from build123d import *

# Parameters (mm, degrees)
SKETCH1_R                = 5
BOSS_EXTRUDE1_DEPTH      = 10
BOSS_EXTRUDE2_DEPTH      = 30
BOSS_EXTRUDE2_DEPTH_BACK = 10
SKETCH2_W                = 140
SKETCH2_H                = 10
CUT_EXTRUDE1_DEPTH       = 30
FILLET1_R                = 10


with BuildPart() as part:
    # Sketch1 → Boss-Extrude1 (new body)
    with BuildSketch(Plane(origin=(0, 0, 0), x_dir=(1, 0, 0), z_dir=(0, 1, 0))):
        with BuildLine():
            Line((0, 0), (0, 35))
            ThreePointArc((0, 35), (4.679111138, 47.855752194), (16.527036447, 54.69615506))
            Line((16.527036447, 54.69615506), (86.139090058, 66.970638294))
            ThreePointArc((86.139090058, 66.970638294), (98.064418846, 65.400638975), (106.932561687, 57.274483234))
            Line((106.932561687, 57.274483234), (140, 0))
            Line((140, 0), (0, 0))
        make_face()
        with Locations(Location((20, 35, 0), (0, 0, 270))):
            Circle(SKETCH1_R, mode=Mode.SUBTRACT)
        with Locations(Location((89.612053611, 47.274483234, 0), (0, 0, 270))):
            Circle(SKETCH1_R, mode=Mode.SUBTRACT)
        with BuildLine():
            Line((122.679491924, 10), (10, 10))
            Line((10, 10), (10, 17.962162855))
            ThreePointArc((10, 17.962162855), (12.003313152, 21.964645576), (16.407947174, 22.759837787))
            ThreePointArc((16.407947174, 22.759837787), (29.771929506, 26.800377555), (31.430453218, 40.662963335))
            ThreePointArc((31.430453218, 40.662963335), (31.448708001, 45.138764747), (35.042512339, 47.806666902))
            Line((35.042512339, 47.806666902), (69.815261378, 53.938040751))
            ThreePointArc((69.815261378, 53.938040751), (74.069509797, 52.692990027), (75.66252141, 48.556434103))
            ThreePointArc((75.66252141, 48.556434103), (83.691884517, 34.57863964), (99.560671411, 37.412543742))
            ThreePointArc((99.560671411, 37.412543742), (103.753425217, 38.851152942), (107.441767577, 36.39251276))
            Line((107.441767577, 36.39251276), (122.679491924, 10))
        make_face(mode=Mode.SUBTRACT)
    extrude(amount=BOSS_EXTRUDE1_DEPTH)

    # Sketch2 → Boss-Extrude2 (add, two sides: drawn at the far end of the back side and taken through both)
    with BuildSketch(Plane(origin=(0, 10, 0), x_dir=(1, 0, 0), z_dir=(0, 1, 0)).offset(-BOSS_EXTRUDE2_DEPTH_BACK)):
        with Locations((70, -5)):
            Rectangle(SKETCH2_W, SKETCH2_H)
    extrude(amount=BOSS_EXTRUDE2_DEPTH + BOSS_EXTRUDE2_DEPTH_BACK)

    # Sketch3 → Cut-Extrude1 (cut)
    with BuildSketch(Plane(origin=(0, 0, 0), x_dir=(-1, 0, 0), z_dir=(0, 0, -1))):
        with BuildLine():
            Line((-125, 31), (-75, 31))
            ThreePointArc((-75, 31), (-69, 25), (-75, 19))
            Line((-75, 19), (-125, 19))
            ThreePointArc((-125, 19), (-131, 25), (-125, 31))
        make_face()
        with BuildLine():
            Line((-55, 31), (-20, 31))
            ThreePointArc((-20, 31), (-14, 25), (-20, 19))
            Line((-20, 19), (-55, 19))
            ThreePointArc((-55, 19), (-61, 25), (-55, 31))
        make_face()
    extrude(amount=-CUT_EXTRUDE1_DEPTH, mode=Mode.SUBTRACT)

    # Fillet1
    fillet1_edges = [part.edges().sort_by_distance(p)[0] for p in [
        (0, 40, 5),
        (140, 40, 5),
    ]]
    fillet(fillet1_edges, radius=FILLET1_R)


solid = part.part
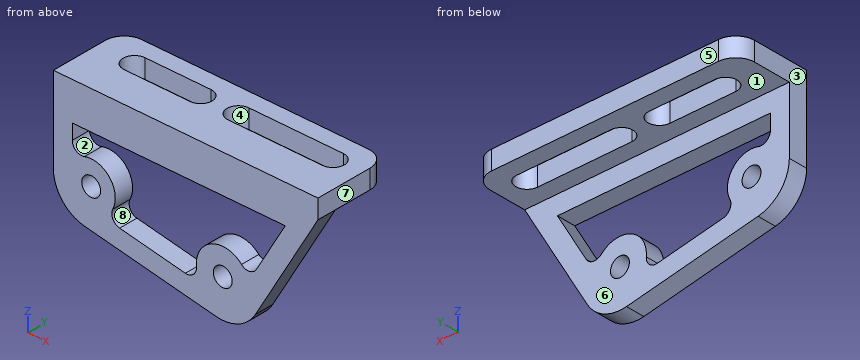
CAD build for the part. Positions are in the model's coordinates, mm. Face numbers are marked on the shaded views. A direction names the side the tool comes from. Round coordinates to 2 decimals unless told otherwise and drop trailing zeros. Write each loop counter-clockwise with the first axis right and the second up, starting at its lowest first coordinate (ties: lowest second). Pieces come first, ordered by that corner, then holes.
(1) Probe line 1 along X through (y, z) = (7, -35); line 2 along Y through (x, z) = (52, 2); line 3 along Y through (x, z) = (17.5, -25). List the from-to ranges inside material, lowest first.
(2) Drop flat-ended pins along their axis: P1, Ø8, axis at x = 60.5, y = 5.5, coming from the -Z side; P2, Ø2, axis at x = 57, z = -56, coming from the +Y side; P3, Ø4, axis at x = 16, y = 9.5, coming from the -Z side. Give the stop position or say it passes through.
(3) Slice it at B-B, the plane x = 58.5. Write the cut outline in (y, z), and give its area (3 significant figures).
(4) 3-axis set-ups, long thin cutter, end or side, ignore diameter. For the marked faces 4, 5, 6, 7 and 8: which of +Z, -Z, +X, -X, +Y, -Y reach the whole face in a straight line?
(5) Mould opens along X. For the marked faces 1, 2 and 3 say: pulls with the +X half, pulls with the -X half, needs draft (parallel to the pull), parting line crosses it, or undercut.
(6) Slice it at D-D, the plane x = 79.5. Write the cut outline in (y, z), and give its area (3 significant figures).
(7) Slice it at C-C, the plane y = 6. Write the cut outline in (x, z), and give its area (3 significant figures).
(8) Slice it at A-A, the plane y = 25. Write the cut outline in (x, z).
From the geometry:
1. line 1: x = 0 to 15, 25 to 32.76, 82.86 to 96.36, 108.25 to 119.79
1. line 2: y = 0 to 19, 31 to 40
1. line 3: y = 0 to 10
2. P1: stops at z = -63.16
2. P2: stops at y = 10
2. P3: stops at z = -54.96
3. outline: (0, -62.1) - (10, -62.1) - (10, -51.94) - (0, -51.94) - close; (0, -10) - (10, -10) - (10, 0) - (20.13, 0) - (20.13, 10) - (0, 10) - close; (29.87, 0) - (40, 0) - (40, 10) - (29.87, 10) - close
3. area: 504 mm2
4. face 4: +Z, -Z
4. face 5: +Z, -Z, +X, -X, +Y
4. face 6: -Z, +X, -X, +Y
4. face 7: +Z, -Z, +X, +Y, -Y
4. face 8: +Y, -Y
5. face 1: needs draft
5. face 2: undercut
5. face 3: pulls with the -X half
6. outline: (0, -65.8) - (10, -65.8) - (10, -37.58) - (0, -37.58) - close; (0, -10) - (10, -10) - (10, 0) - (19, 0) - (19, 10) - (0, 10) - close; (31, 0) - (40, 0) - (40, 10) - (31, 10) - close
6. area: 662 mm2
7. outline: (0, -35) arc R20 ccw to (16.53, -54.7) - (86.14, -66.97) arc R20 ccw to (106.93, -57.27) - (140, 0) - (140, 10) - (0, 10) - close; hole (10, -17.96) arc R5 ccw to (16.41, -22.76) arc R12.76 cw to (31.43, -40.66) arc R5 ccw to (35.04, -47.81) - (69.82, -53.94) arc R5 ccw to (75.66, -48.56) arc R14.01 cw to (99.56, -37.41) arc R5 ccw to (107.44, -36.39) - (122.68, -10) - (10, -10) - close; hole circle Ø10 at (20, -35); hole circle Ø10 at (89.61, -47.27)
7. area: 5,480 mm2
8. outline: (0, 0) - (14, 0) - (14, 10) - (0, 10) - close; (61, 0) - (69, 0) - (69, 10) - (61, 10) - close; (131, 0) - (140, 0) - (140, 10) - (131, 10) - close
